```python
from build123d import *

# Parameters (mm, degrees)
SKETCH1_R                    = 1.5
BOSS_EXTRUDE1_DEPTH          = 6
SALIENTE_EXTRUIR7_DEPTH      = 19
SALIENTE_EXTRUIR7_DEPTH_BACK = 25
CORTAR_EXTRUIR2_DEPTH        = 25
SALIENTE_EXTRUIR8_DEPTH      = 1
SALIENTE_EXTRUIR10_DEPTH     = 1


with BuildPart() as part:
    # Sketch1 → Boss-Extrude1 (new body)
    with BuildSketch(Plane(origin=(0, 0, 0), x_dir=(1, 0, 0), z_dir=(0, 1, 0))):
        with BuildLine():
            Line((0, -5), (23.998875872, -5))
            ThreePointArc((23.998875872, -5), (24.467345461, -4.883479623), (24.826642543, -4.561072489))
            Line((24.826642543, -4.561072489), (28.564941326, 0.954149161))
            ThreePointArc((28.564941326, 0.954149161), (28.766036178, 1.172359953), (29.022312673, 1.321950886))
            Line((29.022312673, 1.321950886), (40.929553216, 6.070049343))
            ThreePointArc((40.929553216, 6.070049343), (41.304486381, 6.141164834), (41.678758689, 6.066649533))
            Line((41.678758689, 6.066649533), (47.144586244, 3.829406729))
            Line((47.144586244, 3.829406729), (48.06174016, 3.086958957))
            Line((48.06174016, 3.086958957), (48.804187932, 4.004112872))
            Line((48.804187932, 4.004112872), (49.721341848, 3.2616651))
            Line((49.721341848, 3.2616651), (50.46378962, 4.178819016))
            Line((50.46378962, 4.178819016), (51.380943536, 3.436371244))
            Line((51.380943536, 3.436371244), (52.123391308, 4.35352516))
            Line((52.123391308, 4.35352516), (53.040545224, 3.611077387))
            Line((53.040545224, 3.611077387), (53.782992996, 4.528231303))
            Line((53.782992996, 4.528231303), (54.700146912, 3.785783531))
            Line((54.700146912, 3.785783531), (55.442594685, 4.702937447))
            Line((55.442594685, 4.702937447), (52.341745918, 12.244834503))
            ThreePointArc((52.341745918, 12.244834503), (52.137055639, 12.558350103), (51.831402108, 12.774604725))
            Line((51.831402108, 12.774604725), (46.024183924, 15.419882568))
            ThreePointArc((46.024183924, 15.419882568), (45.628323444, 15.509674561), (45.229386093, 15.434727162))
            Line((45.229386093, 15.434727162), (20.032711481, 5.075121772))
            ThreePointArc((20.032711481, 5.075121772), (19.846254378, 5.018960187), (19.652448068, 5))
            Line((19.652448068, 5), (0, 5))
            ThreePointArc((0, 5), (-5, 0), (0, -5))
        make_face()
        with Locations(Location((0, 0, 0), (0, 0, 270))):
            Circle(SKETCH1_R, mode=Mode.SUBTRACT)
        with Locations(Location((22, 0, 0), (0, 0, 270))):
            Circle(SKETCH1_R, mode=Mode.SUBTRACT)
    extrude(amount=BOSS_EXTRUDE1_DEPTH)

    # Croquis4 → Saliente-Extruir7 (add, two sides: drawn at the far end of the back side and taken through both)
    with BuildSketch(Plane.XZ.offset(-SALIENTE_EXTRUIR7_DEPTH_BACK)):
        with BuildLine():
            Line((54.700146912, -3.785783531), (55.442594685, -4.702937447))
            Line((55.442594685, -4.702937447), (58.800233779, 3.463526096))
            Line((58.800233779, 3.463526096), (59.114761869, 4.228522601))
            ThreePointArc((59.114761869, 4.228522601), (58.907872463, 4.269394003), (58.700983057, 4.228522601))
            Line((58.700983057, 4.228522601), (53.767339251, -4.508894058))
            Line((53.767339251, -4.508894058), (53.782992996, -4.528231303))
            Line((53.782992996, -4.528231303), (54.700146912, -3.785783531))
        make_face()
        with BuildLine():
            Line((54.16164527, -7.818467854), (54.301219391, -7.478995106))
            Line((54.301219391, -7.478995106), (55.442594685, -4.702937447))
            Line((55.442594685, -4.702937447), (54.700146912, -3.785783531))
            Line((54.700146912, -3.785783531), (53.782992996, -4.528231303))
            Line((53.782992996, -4.528231303), (53.767339251, -4.508894058))
            Line((53.767339251, -4.508894058), (50.221708115, -10.788158993))
            Line((50.221708115, -10.788158993), (40.806466815, -13.616245196))
            Line((40.806466815, -13.616245196), (45.229386093, -15.434727162))
            ThreePointArc((45.229386093, -15.434727162), (45.628323444, -15.509674561), (46.024183924, -15.419882568))
            Line((46.024183924, -15.419882568), (51.831402108, -12.774604725))
            ThreePointArc((51.831402108, -12.774604725), (52.137055639, -12.558350103), (52.341745918, -12.244834503))
            Line((52.341745918, -12.244834503), (54.16164527, -7.818467854))
        make_face()
    extrude(amount=SALIENTE_EXTRUIR7_DEPTH + SALIENTE_EXTRUIR7_DEPTH_BACK)

    # Croquis5 → Cortar-Extruir2 (cut)
    with BuildSketch(Plane.XZ):
        Polygon((41.304486381, -6.141164834), (50.221708115, -10.788158993), (53.767339251, -4.508894058), (53.601046398, -4.303470665), (53.040545224, -3.611077387), (52.123391308, -4.35352516), (51.380943536, -3.436371244), (50.46378962, -4.178819016), (49.721341848, -3.2616651), (48.804187932, -4.004112872), (48.06174016, -3.086958957), (47.144586244, -3.829406729), align=None)
    extrude(amount=-CORTAR_EXTRUIR2_DEPTH, mode=Mode.SUBTRACT)

    # Croquis6 → Saliente-Extruir8 (add)
    with BuildSketch(Plane(origin=(0, -19, 0), x_dir=(-1, 0, 0), z_dir=(0, -1, 0))):
        Polygon((-40.806466815, 13.616245196), (-40.806466815, 0), (-58.700983057, -4.228522601), (-50.221708115, 10.788158993), align=None)
    extrude(amount=-SALIENTE_EXTRUIR8_DEPTH)

    # Croquis7 → Saliente-Extruir10 (add)
    with BuildSketch(Plane(origin=(0, 25, 0), x_dir=(1, 0, 0), z_dir=(0, 1, 0))):
        Polygon((40.806466815, 0), (40.806466815, 13.616245196), (50.221708115, 10.788158993), (58.700983057, -4.228522601), align=None)
    extrude(amount=-SALIENTE_EXTRUIR10_DEPTH)


solid = part.part
```
Could you check a few things on this model? Use its own coordinates, in mm. A direction names the side the tool comes from. Coordinates: 2 decimals unless noted, no trailing zeros. Write each loop counter-clockwise with the first axis right and the second up, starting at its lowest first coordinate (ties: lowest second). Pieces come first, ordered by that corner, then holes. Notation, with made-up numbers: (-36, -39) - (-32, -39) arc R23 ccw to (-32, -25) - close; hole circle Ø7 at (13.25, 79.5). An arc over 180 degrees is marked (long way). Use a Markdown table: item, result.
Q1. Imagine slicing it at A-A (y = 5). List the corners of the cut face in (x, z) for me.
Geometry check:
| item | result |
|---|---|
| outline | (0, -5) - (19.65, -5) arc R1 cw to (20.03, -5.08) - (45.23, -15.43) arc R1 ccw to (46.02, -15.42) - (51.83, -12.77) arc R1 ccw to (52.34, -12.24) - (59.11, 4.23) arc R0.54 ccw to (58.7, 4.23) - (50.22, -10.79) - (41.3, -6.14) arc R1 cw to (40.93, -6.07) - (29.02, -1.32) arc R1 cw to (28.56, -0.95) - (24.83, 4.56) arc R1 ccw to (24, 5) - (0, 5) arc R5 ccw to start; hole circle Ø3 at (0, 0); hole circle Ø3 at (22, 0) |
Q2. Please list where these lines run through material, in increasing order: L1, parallel to Y at x = 45, z = -11; L2, parallel to X at y = 4.7, z = 0; L3, parallel to Y at x = 11, z = 1.25.
Geometry check:
| item | result |
|---|---|
| L1 | y = -19 to -18, 0 to 6, 24 to 25 |
| L2 | x = -5 to -1.5, 1.5 to 20.5, 23.5 to 27.92, 56.31 to 57.38 |
| L3 | y = 0 to 6 |
Q3. Which directions (+Z, -Z, +X, -X, +Y, -Y) give clear straight access to the entire face, cutting with the end or side of a thin tool? Please do faces 4 (the flat face through (48, -18, -5)), 5 (the flat face through (48.887, 3.308, -14.116)), 6 (the flat face through (45.7, 2.96, -8.43)), 7 (the flat face through (26.7, 3, 1.8)).
Geometry check:
| item | result |
|---|---|
| face 4 | +Z, -X |
| face 5 | -Z, +X, +Y, -Y |
| face 6 | +Z |
| face 7 | +Z, +Y, -Y |
Q4. Imagine slicing it at C-C (x = 14). List the corners of the cut face in (y, z) for me.
Geometry check:
| item | result |
|---|---|
| outline | (0, -5) - (6, -5) - (6, 5) - (0, 5) - close |
Q5. Imagine slicing it at B-B (x = 22). List the corners of the cut face in (y, z) for me, and give its area (3 significant figures).
Geometry check:
| item | result |
|---|---|
| outline | (0, -5.88) - (6, -5.88) - (6, -1.5) - (0, -1.5) - close; (0, 1.5) - (6, 1.5) - (6, 5) - (0, 5) - close |
| area | 47.3 mm2 |
Q6. Thinking about a two-plate mould opening in Y: for faces 1 (the flat face through (48, 25, -6)), 2 (the flat face through (45.58, 15.126, -12.182)), 3 (the flat face through (10, 3, -5)), which applies, +Y half, -Y half, draft (parallel to the pull), parting line (faces both ways), or undercut?
Geometry check:
| item | result |
|---|---|
| face 1 | +Y half |
| face 2 | undercut |
| face 3 | draft |
Q7. Imagine slicing it at D-D (x = 30). List the corners of the cut face in (y, z) for me.
Geometry check:
| item | result |
|---|---|
| outline | (0, -9.17) - (6, -9.17) - (6, -1.71) - (0, -1.71) - close |
Q8. I'm going to push flat-ended pins straight in: pin 1 Ø5 at (x, z) = (0, 0) entering from -Y; pin 2 Ø5 at (y, z) = (-6, -3) entering from +X; pin 3 Ø0.8 at (y, z) = (24.5, -8) entering from -X. Where does each tip first touch, or does it pass through?
Geometry check:
| item | result |
|---|---|
| pin 1 | stops at y = 0 |
| pin 2 | stops at x = 57.17 |
| pin 3 | stops at x = 40.81 |
